```python
from build123d import *

# Parameters (mm, degrees)
F2_R = 1.5
F3_R = 4
F4_R = 3


with BuildPart() as f1:
    # F0 (on Front) → F1 (revolve)
    with BuildSketch(Plane.XZ):
        Polygon((0, 55), (0, 0), (24.5, 0), (24.5, 12), (10.5, 20.082904), (13.55485, 55), align=None)
    revolve(axis=Axis((0, 0, 27.5), (0, 0, 1)))

    # F2
    f2_edges = [f1.edges().sort_by_distance(p)[0] for p in [
        (-24.5, 0, 0),
        (-24.5, 0, 12),
    ]]
    fillet(f2_edges, radius=F2_R)

    # F3
    f3_edges = [f1.edges().sort_by_distance(p)[0] for p in [
        (-10.5, 0, 20.082904),
    ]]
    fillet(f3_edges, radius=F3_R)

    # F4
    f4_edges = [f1.edges().sort_by_distance(p)[0] for p in [
        (-13.55485, 0, 55),
    ]]
    fillet(f4_edges, radius=F4_R)


solid = f1.part
```
Geometry: final body of the model. Coordinates: model frame, mm. Round coordinates to 2 decimals unless told otherwise and drop trailing zeros. Write each loop counter-clockwise with the first axis right and the second up, starting at its lowest first coordinate (ties: lowest second). Pieces come first, ordered by that corner, then holes. Notation, with made-up numbers: M 89.5,-17 L 96.5,-17 A20 cw 96.5,3 Z; hole C 19,16.5 d6. An arc over 180 degrees is marked long. Answer in a Markdown table with one row per item. Add a question column.
(1) Contact query for flat-ended pins moving along their axis: pin 1 (10 mm diameter, centred on y = -4, z = 24.5, fed in from +X); pin 2 (12 mm diameter, centred on y = 14, z = 25, fed in from +X); pin 3 (3 mm diameter, centred on y = 7.5, z = 7.5, fed in from -X); pin 4 (1 mm diameter, centred on y = -12.5, z = 35.5, fed in from -X). Output: stop coordinate, or through.
(2) Cut plane B-B, the plane z = 50.5. Return the cut outline in (x, y), then the cut area to 3 significant figures.
(3) Draft query along Z for faces 1 (the face through (0, 0, 0)), 2 (the face through (11.1, -4.6, 37.4)), 3 (the face through (0, 0, 55)). Return one class per face: pulls with the +Z half, pulls with the -Z half, needs draft (parallel to the pull), parting line crosses it, or undercut.
(4) Cut plane A-A, the plane z = 8.5. Return the cut outline in (x, y), then the cut area to 3 significant figures.
(5) Ray query, L1, parallel to Z at x = 7, y = 15.5; L2, parallel to X at y = 8, z = 9; L3, parallel to X at y = 4, z = 10. Return the intervals inside material, ascending.
Established:
| question | item | result |
|---|---|---|
| 1 | pin 1 | x = 11.35 |
| 1 | pin 2 | x = 7.49 |
| 1 | pin 3 | x = -23.75 |
| 1 | pin 4 | through |
| 2 | outline | C 0,0 d26.32 |
| 2 | area | 544 mm² |
| 3 | face 1 | pulls with the -Z half |
| 3 | face 2 | undercut |
| 3 | face 3 | pulls with the +Z half |
| 4 | outline | C 0,0 d49 |
| 4 | area | 1,890 mm² |
| 5 | L1 | 0 to 16.33 |
| 5 | L2 | -23.16 to 23.16 |
| 5 | L3 | -24.17 to 24.17 |
